Source: CAD feature listing. Evaluate the final solid. Frame: model axes, mm. Face numbers are marked on the shaded views. Coordinates: 2 decimals unless noted, no trailing zeros. Write each loop counter-clockwise with the first axis right and the second up, starting at its lowest first coordinate (ties: lowest second). Pieces come first, ordered by that corner, then holes. Notation, with made-up numbers: (6, 71) - (48, 71) arc R18 cw to (48, 87) - close; hole circle Ø1 at (-4.75, 67.25). An arc over 180 degrees is marked (long way). One line per question, with ' | ' between items.
from build123d import *

# Parameters (mm, degrees)
MODEL_R                 = 2.4
SALIENTE_EXTRUIR1_DEPTH = 3


with BuildPart() as part:
    # Model → Saliente-Extruir1 (new body)
    with BuildSketch(Plane.XY):
        with BuildLine():
            Line((0.550846874, 14.545911472), (11.282662542, 21.007019657))
            Line((11.282662542, 21.007019657), (44.011748182, 18.287442361))
            Line((44.011748182, 18.287442361), (43.888957319, 16.809700693))
            ThreePointArc((43.888957319, 16.809700693), (44.855654521, 14.707163158), (47.155246022, 14.448229776))
            Line((47.155246022, 14.448229776), (47.182889346, 14.460182921))
            ThreePointArc((47.182889346, 14.460182921), (47.281916988, 14.506531358), (47.378685576, 14.557428234))
            Line((47.378685576, 14.557428234), (49.127384749, 15.529685066))
            ThreePointArc((49.127384749, 15.529685066), (50.19897968, 15.696696011), (51.122983719, 15.128871311))
            Line((51.122983719, 15.128871311), (51.504698759, 14.677971297))
            ThreePointArc((51.504698759, 14.677971297), (51.91223143, 13.672921311), (51.570646763, 12.643587416))
            Line((51.570646763, 12.643587416), (50.323105233, 11.079339262))
            ThreePointArc((50.323105233, 11.079339262), (50.256934954, 10.992298205), (50.194877883, 10.902278366))
            Line((50.194877883, 10.902278366), (50.178526203, 10.876986992))
            ThreePointArc((50.178526203, 10.876986992), (51.085631167, 7.518902031), (54.34625878, 8.730463665))
            Line((54.34625878, 8.730463665), (54.357353411, 8.758462597))
            ThreePointArc((54.357353411, 8.758462597), (54.394603234, 8.861259009), (54.427039433, 8.965674259))
            Line((54.427039433, 8.965674259), (54.976067079, 10.889680702))
            ThreePointArc((54.976067079, 10.889680702), (55.61570455, 11.765507317), (56.670586767, 12.017364142))
            Line((56.670586767, 12.017364142), (57.259334518, 11.968442975))
            ThreePointArc((57.259334518, 11.968442975), (58.258181294, 11.54593443), (58.744493436, 10.576548618))
            Line((58.744493436, 10.576548618), (58.96843884, 8.588313067))
            ThreePointArc((58.96843884, 8.588313067), (58.983196709, 8.479976292), (59.002969372, 8.372441678))
            Line((59.002969372, 8.372441678), (59.00929069, 8.342995592))
            ThreePointArc((59.00929069, 8.342995592), (62.025235409, 6.609891015), (63.474143857, 9.772206359))
            Line((63.474143857, 9.772206359), (63.462190711, 9.799849683))
            ThreePointArc((63.462190711, 9.799849683), (63.415842275, 9.898877325), (63.364945399, 9.995645912))
            Line((63.364945399, 9.995645912), (62.392688567, 11.744345086))
            ThreePointArc((62.392688567, 11.744345086), (62.225677622, 12.815940017), (62.793502322, 13.739944056))
            Line((62.793502322, 13.739944056), (63.244402336, 14.121659096))
            ThreePointArc((63.244402336, 14.121659096), (64.249452322, 14.529191767), (65.278786217, 14.187607099))
            Line((65.278786217, 14.187607099), (66.843034372, 12.940065573))
            ThreePointArc((66.843034372, 12.940065573), (66.930075429, 12.873895294), (67.020095268, 12.811838223))
            Line((67.020095268, 12.811838223), (67.045386643, 12.795486542))
            ThreePointArc((67.045386643, 12.795486542), (70.403471604, 13.702591507), (69.191909969, 16.963219119))
            Line((69.191909969, 16.963219119), (69.163911037, 16.974313751))
            ThreePointArc((69.163911037, 16.974313751), (69.061114626, 17.011563574), (68.956699375, 17.043999773))
            Line((68.956699375, 17.043999773), (67.107784068, 17.571599676))
            ThreePointArc((67.107784068, 17.571599676), (60.941730208, 29.535754633), (48.612503883, 24.136550776))
            Line((48.612503883, 24.136550776), (11.796901511, 27.195691428))
            Line((11.796901511, 27.195691428), (-2.378510761, 19.779467823))
            ThreePointArc((-2.378510761, 19.779467823), (-3.605636909, 15.656016384), (0.550846874, 14.545911472))
        make_face()
        with Locations((57.652706647, 20.269666987)):
            Circle(MODEL_R, mode=Mode.SUBTRACT)
    extrude(amount=SALIENTE_EXTRUIR1_DEPTH)


solid = part.part
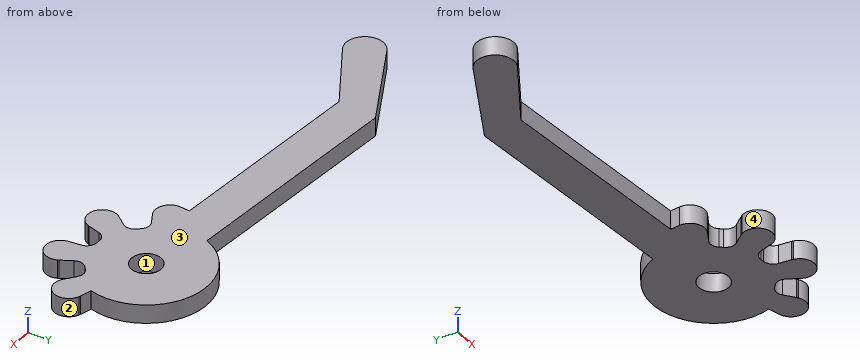
Item 1: Cut plane A-A on y = 22. Return loops of the section in (x, z).
Check sheet entries:
outline: (1.87, 0) - (55.99, 0) - (55.99, 3) - (1.87, 3) - close; (59.32, 0) - (67.33, 0) - (67.33, 3) - (59.32, 3) - close
Item 2: Mould query, pull axis Y, two halves, no side actions, for the marked faces 1, 2, 3 and 4. Classes: pulls with the +Y half, pulls with the -Y half, needs draft (parallel to the pull), parting line crosses it, or undercut.
Check sheet entries:
face 1: undercut | face 2: parting line crosses it | face 3: needs draft | face 4: undercut
Item 3: Cut plane C-C on x = 23.5. Return loops of the section in (y, z), and give its area (3 significant figures).
Check sheet entries:
outline: (19.99, 0) - (26.22, 0) - (26.22, 3) - (19.99, 3) - close | area: 18.7 mm²
Item 4: Pin query (flat end, axial travel): pin 1 Ø1.5 at (x, z) = (20, 1) entering from +Y; pin 2 Ø1.5 at (x, y) = (26.5, 19.5) entering from +Z. Return the tip coordinate at first contact, or that it passes through.
Check sheet entries:
pin 1: y = 26.58 | pin 2: z = 3
Item 5: Cut plane B-B on y = 26.5. Return loops of the section in (x, z), and give its area (3 significant figures).
Check sheet entries:
outline: (10.47, 0) - (20.17, 0) - (20.17, 3) - (10.47, 3) - close; (50.05, 0) - (65.26, 0) - (65.26, 3) - (50.05, 3) - close | area: 74.7 mm²
Item 6: Ray query, line 1 along X through (y, z) = (8.25, 2.25); line 2 along X through (y, z) = (16, 0.4); line 3 along X through (y, z) = (28.25, 0.6). Return the intervals inside material, ascending. Write a range as [from, to].
Check sheet entries:
line 1: [50.24, 54.08], [59.03, 63.58] | line 2: [-3.77, 2.97], [43.96, 70.32] | line 3: [51.91, 63.4]
Item 7: Cut plane D-D on x = 8. Return loops of the section in (y, z).
Check sheet entries:
outline: (19.03, 0) - (25.21, 0) - (25.21, 3) - (19.03, 3) - close
